Here's how the part is built. I have some questions about the finished solid (model axes, mm). Face numbers are marked on the shaded views. A direction names the side the tool comes from. Give positions to 0.01 mm unless a question says otherwise; leave off trailing zeros. Write each loop counter-clockwise with the first axis right and the second up, starting at its lowest first coordinate (ties: lowest second). Pieces come first, ordered by that corner, then holes. Notation, with made-up numbers: M 68.25,27.5 L 81.25,27.5 A24 ccw 81.25,59.5 Z; hole C -9,15.5 d6. An arc over 180 degrees is marked long. Answer as CSV lines item,"result". Start each with the question number.
Q1. Thinking about a two-plate mould opening in Y: for the marked faces 3, 4 and 5, which applies, +Y half, -Y half, draft (parallel to the pull), parting line (faces both ways), or undercut?
Q2. Suppose I cut it at B-B (x = 31.75). Write out the boundary of the cut face in (y, z) (1 decimal).
Q3. Suppose I cut it at D-D (x = 85.5). Write out the boundary of the cut face in (y, z) (1 decimal), then the cut area to 3 significant figures.
Q4. If I drill on line 1 along X through (y, z) = (2, 44); line 2 along X through (y, z) = (44, 4); line 3 along Y through (x, z) = (13, 20.5), over which ranges is the centre line in solid material (lowest first)?
Q5. On a 3-axis mill with a long thin cutter (end or side, diameter ignored), from which of +Z, -Z, +X, -X, +Y, -Y can I reach the whole of each face in a straight line? I mean the marked faces 1 and 2. Say none if no direction works.
Q6. Suppose I cut it at A-A (z = 16.5). Write out the boundary of the cut face in (x, y), then the cut area to 3 significant figures.
Q7. Suppose I cut it at C-C (y = 44.45). Write out the boundary of the cut face in (x, z), then the cut area to 3 significant figures.
Q8. For pin 1 (12 mm diameter, centred on x = 34.5, y = 41.5, fed in from +Z); pin 2 (17.5 mm diameter, centred on y = 6, z = 18.5, fed in from +X); pin 3 (4 mm diameter, centred on y = 31.5, z = 8, fed in from +X), each with a flat end and sliding along its axis, tell me the tip position at first contact or that it passes through.
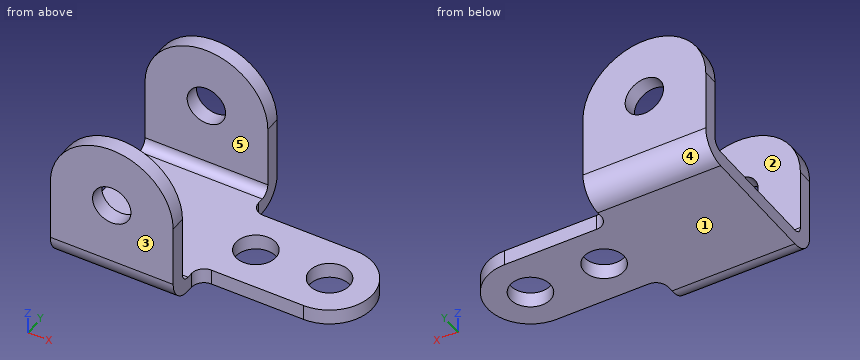
```python
from build123d import *

# Parameters (mm, degrees)
F0_R     = 10.3251
F2_DEPTH = 7.9375
F1_R     = 9.92251
F3_DEPTH = 88.9
F4_W     = 73.025
F4_H     = 76.2
F5_DEPTH = 63.501
F6_R     = 12.7
F7_R     = 4.7625


with BuildPart() as f2:
    # F0 (on Top) → F2 (new body)
    with BuildSketch(Plane.XY):
        with BuildLine():
            Line((0, 88.9), (0, 0))
            Line((0, 0), (63.5, 0))
            Line((63.5, 0), (63.5, 15.875))
            ThreePointArc((63.5, 15.875), (65.359872, 20.365128), (69.85, 22.225))
            Line((69.85, 22.225), (117.475, 22.225))
            ThreePointArc((117.475, 22.225), (139.7, 44.45), (117.475, 66.675))
            Line((117.475, 66.675), (69.85, 66.675))
            ThreePointArc((69.85, 66.675), (65.359872, 68.534872), (63.5, 73.025))
            Line((63.5, 73.025), (63.5, 88.9))
            Line((63.5, 88.9), (0, 88.9))
        make_face()
        with Locations((79.375, 44.45)):
            Circle(F0_R, mode=Mode.SUBTRACT)
        with Locations((117.475, 44.45)):
            Circle(F0_R, mode=Mode.SUBTRACT)
    extrude(amount=F2_DEPTH)

    # F1 (on Front) → F3 (join)
    with BuildSketch(Plane.XZ):
        with BuildLine():
            Line((0, 44.45), (0, 0))
            Line((0, 0), (63.5, 0))
            Line((63.5, 0), (63.5, 44.45))
            ThreePointArc((63.5, 44.45), (31.75, 76.2), (0, 44.45))
        make_face()
        with Locations((31.75, 44.45)):
            Circle(F1_R, mode=Mode.SUBTRACT)
    extrude(amount=-F3_DEPTH)

    # F4 (on face) → F5 (cut, through all)
    with BuildSketch(Plane.YZ.offset(63.5)):
        with Locations((44.45, 46.0375)):
            Rectangle(F4_W, F4_H)
    extrude(amount=-F5_DEPTH, mode=Mode.SUBTRACT)

    # F6
    f6_edges = [f2.edges().sort_by_distance(p)[0] for p in [
        (31.75, 0, 0),
        (31.75, 88.9, 0),
    ]]
    fillet(f6_edges, radius=F6_R)

    # F7
    f7_edges = [f2.edges().sort_by_distance(p)[0] for p in [
        (31.75, 7.9375, 7.9375),
        (31.75, 80.9625, 7.9375),
    ]]
    fillet(f7_edges, radius=F7_R)


solid = f2.part
```
Resolved:
1,face 3,"-Y half"
1,face 4,"+Y half"
1,face 5,"undercut"
2,outline,"M 0,12.7 A12.7 ccw 12.7,0 L 76.2,0 A12.7 ccw 88.9,12.7 L 88.9,34.5 L 81,34.5 L 81,12.7 A4.8 cw 76.2,7.9 L 12.7,7.9 A4.8 cw 7.9,12.7 L 7.9,34.5 L 0,34.5 Z; M 0,54.4 L 7.9,54.4 L 7.9,76.2 L 0,76.2 Z; M 81,54.4 L 88.9,54.4 L 88.9,76.2 L 81,76.2 Z"
3,outline,"M 22.2,0 L 36.1,0 L 36.1,7.9 L 22.2,7.9 Z; M 52.8,0 L 66.7,0 L 66.7,7.9 L 52.8,7.9 Z"
3,area,"221 mm^2"
4,line 1,"0 to 21.84, 41.66 to 63.5"
4,line 2,"0 to 69.06, 89.69 to 107.16, 127.79 to 139.7"
4,line 3,"0 to 7.94, 80.96 to 88.9"
5,face 1,"-Z, +X, -X, +Y, -Y"
5,face 2,"+Z, +X, -X"
6,outline,"M 0,0 L 63.5,0 L 63.5,7.94 L 0,7.94 Z; M 0,80.96 L 63.5,80.96 L 63.5,88.9 L 0,88.9 Z"
6,area,"1,010 mm^2"
7,outline,"M 0,0 L 69.05,0 L 69.05,7.94 L 0,7.94 Z; M 89.7,0 L 107.15,0 L 107.15,7.94 L 89.7,7.94 Z; M 127.8,0 L 139.7,0 L 139.7,7.94 L 127.8,7.94 Z"
7,area,"781 mm^2"
8,pin 1,"z = 7.94"
8,pin 2,"x = 63.5"
8,pin 3,"x = 136.81"
